Autodesk Fusion 360 part; units mm, degrees
sketch "Sketch1" plane through (0, 0, 0) normal (1, 0, 0) x (0, 1, 0)
  line L0 (-31.75, 0) -> (31.75, 0) construction
  line L1 (-31.75, 0) -> (-31.75, 1.7)
  line L2 (31.75, 0) -> (31.75, 1.7)
  line L3 (0, 0) -> (0, 8.4) construction
  line L4 (-5.65, 8.4) -> (5.65, 8.4) construction
  line L5 (-10.65, 8.4) -> (10.65, 8.4) construction
  line L6 (-5.65, 8.4) -> (-10.65, 8.4)
  line L7 (5.65, 8.4) -> (10.65, 8.4)
  line L8 (-17.5, 1.7) -> (17.5, 1.7) construction
  line L9 (-31.75, 1.7) -> (-17.5, 1.7)
  line L10 (-17.5, 1.7) -> (-10.65, 8.4)
  line L11 (31.75, 1.7) -> (17.5, 1.7)
  line L12 (17.5, 1.7) -> (10.65, 8.4)
  line L13 (-30.05, 0) -> (-16.8068, 0)
  line L14 (-16.8068, 0) -> (-9.9568, 6.7)
  line L15 (-5.65, 6.7) -> (-9.9568, 6.7)
  line L16 (30.05, 0) -> (16.8068, 0)
  line L17 (16.8068, 0) -> (9.9568, 6.7)
  line L18 (5.65, 6.7) -> (9.9568, 6.7)
  line L19 (-5.65, 6.7) -> (-5.65, 8.4)
  line L20 (5.65, 6.7) -> (5.65, 8.4)
  line L21 (-30.05, 0) -> (-31.75, 0)
  line L22 (30.05, 0) -> (31.75, 0)
  dimension "d1" = 63.5
  dimension "d2" = 1.7
  dimension "d3" = 1.7
  dimension "d4" = 8.4
  dimension "d5" = 11.3
  dimension "d6" = 21.3
  dimension "d7" = 5
  dimension "d8" = 5
  dimension "d9" = 35
  dimension "d10" = 1.7
  dimension "d11" = -1.7
revolve "Revolve1" add sketch "Sketch1" angle 360 about axis through (0, 0, 0) along (0, 0, 1) contours L1 L6 L9 L10 L13 L14 L15 L19 L21
sketch "Sketch2" plane through (0, 0, 0) normal (0, 0, -1) x (1, 0, 0)
  circle A0 centre (0, 0) radius 16.8068
  circle A1 centre (0, 0) radius 31.75
  line L0 (0.5, -31.75) -> (-0.5, -31.75)
  line L1 (-0.5, -31.75) -> (-0.5, -23.25)
  line L2 (-0.5, -23.25) -> (0.5, -23.25)
  line L3 (0.5, -23.25) -> (0.5, -31.75)
  circle A2 centre (0, 0) radius 31.75
  line L4 (0, -31.75) -> (0, 31.75) construction
  dimension "d13" = 1
  dimension "d14" = 8.5
  dimension "d15" = 63.5
extrude "Extrude1" cut sketch "Sketch2" against normal blind 0.4 contours A1 L1 L2 L3 A2 picked at (0, -26.0833)
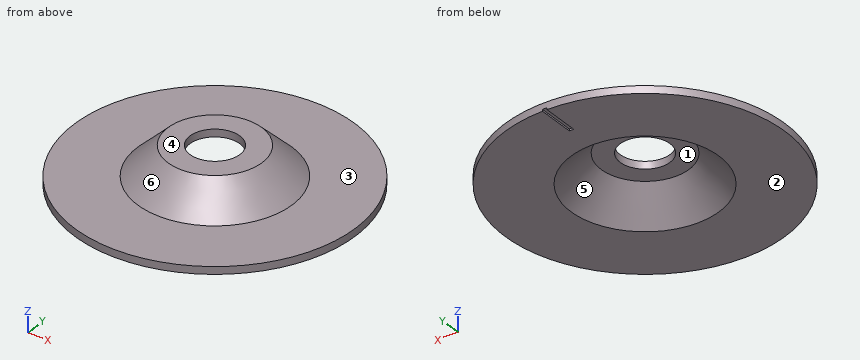
Geometry: final body of the model. Coordinates: model frame, mm. Face numbers are marked on the shaded views. A direction names the side the tool comes from. Give positions to 0.01 mm unless a question says otherwise; leave off trailing zeros. Loops run counter-clockwise (first coordinate to the right, second up) from the corner with the lowest first, then second, coordinate; pieces in that order, holes last. Notation, with made-up numbers: (-13.5, 45) -> (17.5, 45) arc R12 ccw to (17.5, 50) -> close; hole circle Ø8 at (-24, -24.75). An arc over 180 degrees is marked (long way). Return JSON: item names as keys, results as strings.
Item 1: Access query for the marked faces 1, 2 and 3. Directions: +Z, -Z, +X, -X, +Y, -Y. A direction counts if a zero-diameter tool reaches every point of the face in a straight line with its end or side. Return the directions, or none.
Filled in:
{"face 1": "-Z", "face 2": "-Z, +X, -X, +Y, -Y", "face 3": "+Z"}
Item 2: Pin query (flat end, axial travel): P1, Ø2, axis at x = 2, y = 17.5, coming from the -Z side; P2, Ø3, axis at y = 14.5, z = 3.5, coming from the -X side; P3, Ø1, axis at x = 10.5, z = 5.5, coming from the +Y side; P4, Ø8, axis at x = -1.5, y = 19, coming from the +Z side. Return the tip coordinate at first contact, or that it passes through.
Filled in:
{"P1": "z = 0", "P2": "x = -10.01", "P3": "y = 9.62", "P4": "z = 4.09"}
Item 3: Mould query, pull axis X, two halves, no side actions, for the marked faces 4, 5 and 6. Classes: released by +X, released by -X, zero draft, split by the parting line, or undercut.
Filled in:
{"face 4": "zero draft", "face 5": "undercut", "face 6": "split by the parting line"}
Item 4: Section D-D, the plane x = 26. Output: boundary loops of the cut face in (y, z).
Filled in:
{"outline": "(-18.22, 0) -> (18.22, 0) -> (18.22, 1.7) -> (-18.22, 1.7) -> close"}
Item 5: Section C-C, the plane y = 24.5. Output: boundary loops of the cut face in (x, z).
Filled in:
{"outline": "(-20.19, 0) -> (-0.5, 0) -> (-0.5, 0.4) -> (0.5, 0.4) -> (0.5, 0) -> (20.19, 0) -> (20.19, 1.7) -> (-20.19, 1.7) -> close"}
Item 6: Line query: line 1 (Z direction, x = -16.5, y = -21.5); line 2 (X direction, y = 0, z = 7.9); line 3 (X direction, y = 0, z = 7.2). Output: solid intervals per line, ascending.
Filled in:
{"line 1": "0 to 1.7", "line 2": "-11.16 to -5.65, 5.65 to 11.16", "line 3": "-11.88 to -5.65, 5.65 to 11.88"}
Item 7: Section A-A, the plane y = 0. Output: boundary loops of the cut face in (x, z).
Filled in:
{"outline": "(-31.75, 0) -> (-16.81, 0) -> (-9.96, 6.7) -> (-5.65, 6.7) -> (-5.65, 8.4) -> (-10.65, 8.4) -> (-17.5, 1.7) -> (-31.75, 1.7) -> close; (5.65, 6.7) -> (9.96, 6.7) -> (16.81, 0) -> (31.75, 0) -> (31.75, 1.7) -> (17.5, 1.7) -> (10.65, 8.4) -> (5.65, 8.4) -> close"}
Item 8: Section B-B, the plane z = 7.5. Output: boundary loops of the cut face in (x, y), plus the area to 3 significant figures.
Filled in:
{"outline": "circle Ø23.14 at (0, 0); hole circle Ø11.3 at (0, 0)", "area": "320 mm^2"}
